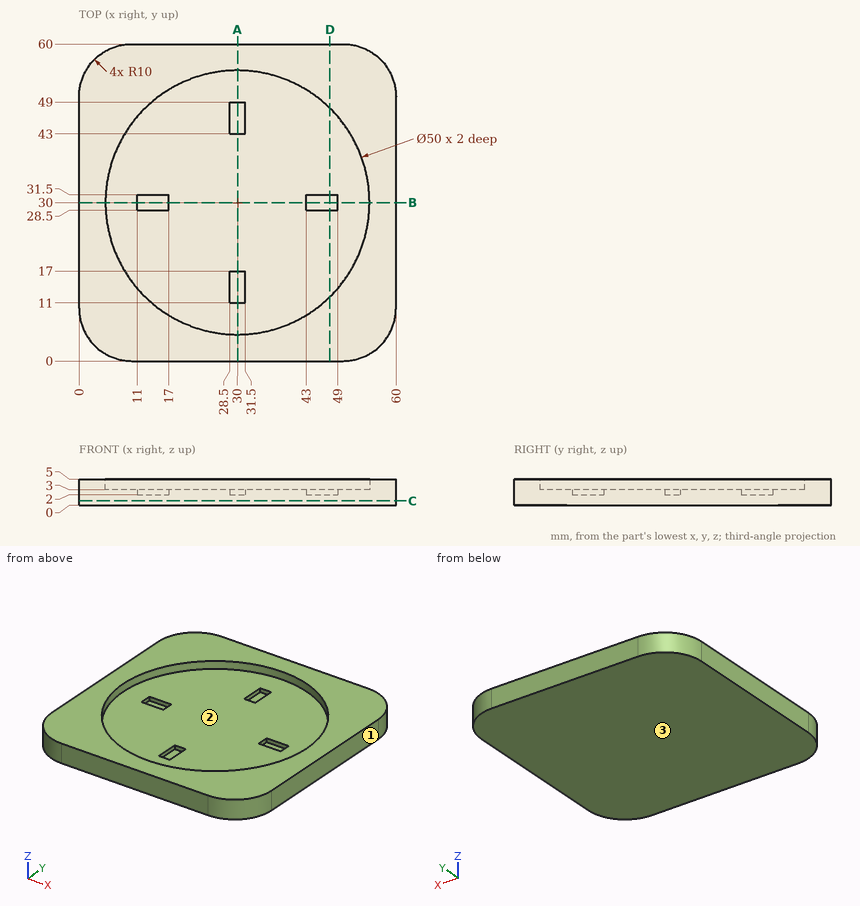
Verification items for this drawing (mm, ordinates from the low corner). Give positions to 0.01 mm unless a question says otherwise; leave off trailing zeros. Write each loop counter-clockwise with the first axis right and the second up, starting at its lowest first coordinate (ties: lowest second). Pieces come first, ordered by that corner, then holes. Notation, with made-up numbers: (79, 78) -> (122, 78) arc R32 ccw to (122, 106) -> close; hole circle Ø11 at (68, 73.25). An arc over 180 degrees is marked (long way). Write item = value, one per line.
Item 1: Sectioned sample at A-A on x = 30. Record the boundary of the cut face in (y, z), and give its area (3 significant figures).
Output:
outline = (0, 0) -> (60, 0) -> (60, 5) -> (55, 5) -> (55, 3) -> (49, 3) -> (49, 2) -> (43, 2) -> (43, 3) -> (17, 3) -> (17, 2) -> (11, 2) -> (11, 3) -> (5, 3) -> (5, 5) -> (0, 5) -> close
area = 188 mm^2
Item 2: Sectioned sample at D-D on x = 47.5. Record the boundary of the cut face in (y, z).
Output:
outline = (0, 0) -> (60, 0) -> (60, 5) -> (47.85, 5) -> (47.85, 3) -> (31.5, 3) -> (31.5, 2) -> (28.5, 2) -> (28.5, 3) -> (12.15, 3) -> (12.15, 5) -> (0, 5) -> close
Item 3: Sectioned sample at C-C on z = 0.85. Record the boundary of the cut face in (x, y).
Output:
outline = (0, 10) arc R10 ccw to (10, 0) -> (50, 0) arc R10 ccw to (60, 10) -> (60, 50) arc R10 ccw to (50, 60) -> (10, 60) arc R10 ccw to (0, 50) -> close
Item 4: Release check for a two-part mould opening along X. For the marked faces 1, 2 and 3 record: +X half, -X half, draft (parallel to the pull), parting line (faces both ways), or undercut.
Output:
face_1 = +X half
face_2 = undercut
face_3 = draft
Item 5: Scan lines: probe 1 along X at (y, z) = (12.5, 2.25); probe 2 along Y at (x, z) = (30, 4.2); probe 3 along Z at (x, y) = (22, 8). Record each from-to range of solid material in increasing order. Write a range as from..to.
Output:
probe_1 = 0..28.5, 31.5..60
probe_2 = 0..5, 55..60
probe_3 = 0..3
Item 6: Gauge pin test, flat ends, axial feed: pin 1 (3 mm diameter, centred on x = 33.5, y = 48, fed in from +Z); pin 2 (0.9 mm diameter, centred on x = 13.5, y = 30.5, fed in from +Z). Record the tip position at first contact, or that the pin passes through.
Output:
pin_1 = 3
pin_2 = 2
